Read the model definition and answer for the solid it produces. Units are mm, in the model's axes. Face numbers are marked on the shaded views. A direction names the side the tool comes from. Coordinates: 2 decimals unless noted, no trailing zeros. Write each loop counter-clockwise with the first axis right and the second up, starting at its lowest first coordinate (ties: lowest second). Pieces come first, ordered by that corner, then holes. Notation, with made-up numbers: (-15.5, 28) -> (-6.5, 28) arc R6 cw to (-6.5, 34) -> close; hole circle Ø9 at (39, -26.75). An arc over 180 degrees is marked (long way). One line per item, written item: value. Start each with the question number.
1. Find section B-B, the plane z = -224.5. Write down the section's boundary in (x, y).
2. Given P1, Ø10, axis at x = -202, y = 353, coming from the +Z side; P2, Ø6, axis at x = -150.5, y = -49, coming from the -Z side; P3, Ø5, axis at x = -304, y = -200.5, coming from the +Z side, each flat-ended and moving along its own axis, determine where each tip first touches the part or whether it passes through.
3. Consider line 1 along X through (y, z) = (336.5, 90); line 2 along X through (y, z) = (-160, 61); line 3 along Z through (x, y) = (272, 429.5). Determine where each line is inside the solid, lowest interval first.
4. For a pull along X with two mould halves and no side action, classify the marked faces 4, 5, 6 and 7 as pulls with the +X half, pulls with the -X half, needs draft (parallel to the pull), parting line crosses it, or undercut.
5. Find section C-C, the plane x = -54. Write down the section's boundary in (y, z).
6. Find section A-A, the plane y = -318. Write down the section's boundary in (x, z).
7. For the marked faces 1, 2 and 3, determine the directions among +Z, -Z, +X, -X, +Y, -Y from which every point of the face is accessible in a straight line to the end or side of a thin tool.
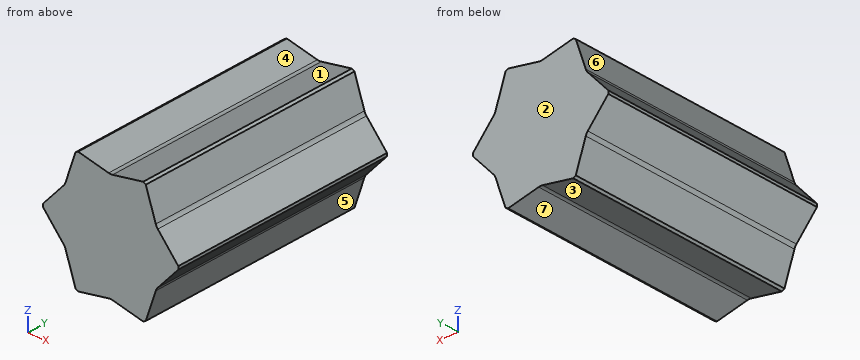
```python
from build123d import *

# Parameters (mm, degrees)
EXTRUDE_1_DEPTH          = 660
CUT_EXTRUDE_1_DEPTH      = 661
CUT_EXTRUDE_1_DEPTH_BACK = 661


with BuildPart() as part:
    # 草图1 → 凸台-拉伸1 (new body, symmetric)
    with BuildSketch(Plane(origin=(0, 0, 0), x_dir=(1, 0, 0), z_dir=(0, 1, 0))):
        Polygon((395, 8.660254038), (205, 337.749907476), (190, 346.410161514), (-190, 346.410161514), (-205, 337.749907476), (-395, 8.660254038), (-395, -8.660254038), (-205, -337.749907476), (-190, -346.410161514), (190, -346.410161514), (205, -337.749907476), (395, -8.660254038), align=None)
    extrude(amount=EXTRUDE_1_DEPTH, both=True)

    # 草图4 → 切除-拉伸1 (cut, two sides)
    with BuildSketch(Plane(origin=(0, 0, 0), x_dir=(1, 0, 0), z_dir=(0, 1, 0))) as cut_extrude_1_sk:
        with BuildLine():
            Line((190, 369.620348729), (190, 346.410161514))
            Line((190, 346.410161514), (11.76, 310.784114995))
            ThreePointArc((11.76, 310.784114995), (0, 309.620348729), (-11.76, 310.784114995))
            Line((-11.76, 310.784114995), (-190, 346.410161514))
            Line((-190, 346.410161514), (-190, 369.620348729))
            Line((-190, 369.620348729), (-190, 392.830535944))
            Line((-190, 392.830535944), (-11.76, 428.456582463))
            ThreePointArc((-11.76, 428.456582463), (0, 429.620348729), (11.76, 428.456582463))
            Line((11.76, 428.456582463), (190, 392.830535944))
            Line((190, 392.830535944), (190, 369.620348729))
        make_face()
        with BuildLine():
            Line((415.100611755, 20.265347645), (395, 8.660254038))
            Line((395, 8.660254038), (275.026938678, 145.207598749))
            ThreePointArc((275.026938678, 145.207598749), (268.139087528, 154.810174364), (263.266938678, 165.576516246))
            Line((263.266938678, 165.576516246), (205, 337.749907476))
            Line((205, 337.749907476), (225.100611755, 349.355001084))
            Line((225.100611755, 349.355001084), (245.20122351, 360.960094691))
            Line((245.20122351, 360.960094691), (365.174284832, 224.41274998))
            ThreePointArc((365.174284832, 224.41274998), (372.062135982, 214.810174364), (376.934284832, 204.043832483))
            Line((376.934284832, 204.043832483), (435.20122351, 31.870441253))
            Line((435.20122351, 31.870441253), (415.100611755, 20.265347645))
        make_face()
        with BuildLine():
            Line((225.100611755, -349.355001084), (205, -337.749907476))
            Line((205, -337.749907476), (263.266938678, -165.576516246))
            ThreePointArc((263.266938678, -165.576516246), (268.139087528, -154.810174364), (275.026938678, -145.207598749))
            Line((275.026938678, -145.207598749), (395, -8.660254038))
            Line((395, -8.660254038), (415.100611755, -20.265347645))
            Line((415.100611755, -20.265347645), (435.20122351, -31.870441253))
            Line((435.20122351, -31.870441253), (376.934284832, -204.043832483))
            ThreePointArc((376.934284832, -204.043832483), (372.062135982, -214.810174364), (365.174284832, -224.41274998))
            Line((365.174284832, -224.41274998), (245.20122351, -360.960094691))
            Line((245.20122351, -360.960094691), (225.100611755, -349.355001084))
        make_face()
        with BuildLine():
            Line((-190, -369.620348729), (-190, -346.410161514))
            Line((-190, -346.410161514), (-11.76, -310.784114995))
            ThreePointArc((-11.76, -310.784114995), (0, -309.620348729), (11.76, -310.784114995))
            Line((11.76, -310.784114995), (190, -346.410161514))
            Line((190, -346.410161514), (190, -369.620348729))
            Line((190, -369.620348729), (190, -392.830535944))
            Line((190, -392.830535944), (11.76, -428.456582463))
            ThreePointArc((11.76, -428.456582463), (0, -429.620348729), (-11.76, -428.456582463))
            Line((-11.76, -428.456582463), (-190, -392.830535944))
            Line((-190, -392.830535944), (-190, -369.620348729))
        make_face()
        with BuildLine():
            Line((-415.100611755, -20.265347645), (-395, -8.660254038))
            Line((-395, -8.660254038), (-275.026938678, -145.207598749))
            ThreePointArc((-275.026938678, -145.207598749), (-268.139087528, -154.810174364), (-263.266938678, -165.576516246))
            Line((-263.266938678, -165.576516246), (-205, -337.749907476))
            Line((-205, -337.749907476), (-225.100611755, -349.355001084))
            Line((-225.100611755, -349.355001084), (-245.20122351, -360.960094691))
            Line((-245.20122351, -360.960094691), (-365.174284832, -224.41274998))
            ThreePointArc((-365.174284832, -224.41274998), (-372.062135982, -214.810174364), (-376.934284832, -204.043832483))
            Line((-376.934284832, -204.043832483), (-435.20122351, -31.870441253))
            Line((-435.20122351, -31.870441253), (-415.100611755, -20.265347645))
        make_face()
        with BuildLine():
            Line((-225.100611755, 349.355001084), (-205, 337.749907476))
            Line((-205, 337.749907476), (-263.266938678, 165.576516246))
            ThreePointArc((-263.266938678, 165.576516246), (-268.139087528, 154.810174364), (-275.026938678, 145.207598749))
            Line((-275.026938678, 145.207598749), (-395, 8.660254038))
            Line((-395, 8.660254038), (-415.100611755, 20.265347645))
            Line((-415.100611755, 20.265347645), (-435.20122351, 31.870441253))
            Line((-435.20122351, 31.870441253), (-376.934284832, 204.043832483))
            ThreePointArc((-376.934284832, 204.043832483), (-372.062135982, 214.810174364), (-365.174284832, 224.41274998))
            Line((-365.174284832, 224.41274998), (-245.20122351, 360.960094691))
            Line((-245.20122351, 360.960094691), (-225.100611755, 349.355001084))
        make_face()
    extrude(amount=CUT_EXTRUDE_1_DEPTH, mode=Mode.SUBTRACT)
    extrude(cut_extrude_1_sk.sketch, amount=-CUT_EXTRUDE_1_DEPTH_BACK, mode=Mode.SUBTRACT)


solid = part.part
```
Answer block:
1. outline: (-243.33, -660) -> (243.33, -660) -> (243.33, 660) -> (-243.33, 660) -> close
2. P1: stops at z = 342.37
2. P2: stops at z = -339.11
2. P3: stops at z = 115.08
3. line 1: x = -323.53 to 323.53
3. line 2: x = -349.01 to 349.01
3. line 3: z = -148.94 to 148.94
4. face 4: undercut
4. face 5: pulls with the +X half
4. face 6: pulls with the -X half
4. face 7: undercut
5. outline: (-660, -319.23) -> (660, -319.23) -> (660, 319.23) -> (-660, 319.23) -> close
6. outline: (-395, -8.66) -> (-275.03, -145.21) arc R60 cw to (-263.27, -165.58) -> (-205, -337.75) -> (-190, -346.41) -> (-11.76, -310.78) arc R60 cw to (11.76, -310.78) -> (190, -346.41) -> (205, -337.75) -> (263.27, -165.58) arc R60 cw to (275.03, -145.21) -> (395, -8.66) -> (395, 8.66) -> (275.03, 145.21) arc R60 cw to (263.27, 165.58) -> (205, 337.75) -> (190, 346.41) -> (11.76, 310.78) arc R60 cw to (-11.76, 310.78) -> (-190, 346.41) -> (-205, 337.75) -> (-263.27, 165.58) arc R60 cw to (-275.03, 145.21) -> (-395, 8.66) -> close
7. face 1: +Z, +Y, -Y
7. face 2: +Z, -Z, +X, -X, +Y
7. face 3: -Z, +Y, -Y
